The figure shows three views and two pictorial views of one solid part (mm, origin at its lowest corner). Answer the questions. A direction names the side the tool comes from. Coordinates: 2 decimals unless noted, no trailing zeros. Write each loop counter-clockwise with the first axis right and the second up, starting at its lowest first coordinate (ties: lowest second). Pieces come first, ordered by that corner, then holes. Notation, with made-up numbers: (41, 46) - (54, 46) arc R20 ccw to (54, 68) - close; hole circle Ø3 at (16, 4.25). An arc over 180 degrees is marked (long way). Use a Markdown table: item, result. Add a question column.
(1) The part is cut by section B-B, the plane y = 10. Give the vertices of the cut face in (x, z), then the cut area to 3 significant figures.
(2) The part is cut by section D-D, the plane y = 2.75. Give the vertices of the cut face in (x, z), then the cut area to 3 significant figures.
(3) For a pull along X with two mould halves and no side action, classify the marked faces 1, 2 and 3 as released by +X, released by -X, zero draft, split by the parting line, or undercut.
(4) A tool of negligible diameter and unlimited length cuts with its end or side. For the marked faces 4 and 5, from which of +Z, -Z, +X, -X, +Y, -Y can it reach the whole face along a straight path? Write none if from no direction.
(5) Find the intervals of material crossed by line 1 (Y direction, x = 3.5, z = 1.75); line 2 (Y direction, x = 10, z = 1.4); line 3 (X direction, y = 9.25, z = 1.9), in increasing order. Write a range as from..to.
(6) Given pin 1 Ø10 at (x, y) = (6, 12) entering from +Z; pin 2 Ø1 at (y, z) = (14.5, 1.5) entering from -X, each flat-ended and moving along its own axis, determine where each tip first touches the part or whether it passes through.
(7) The part is cut by section A-A, the plane z = 1.75. Give the vertices of the cut face in (x, y).
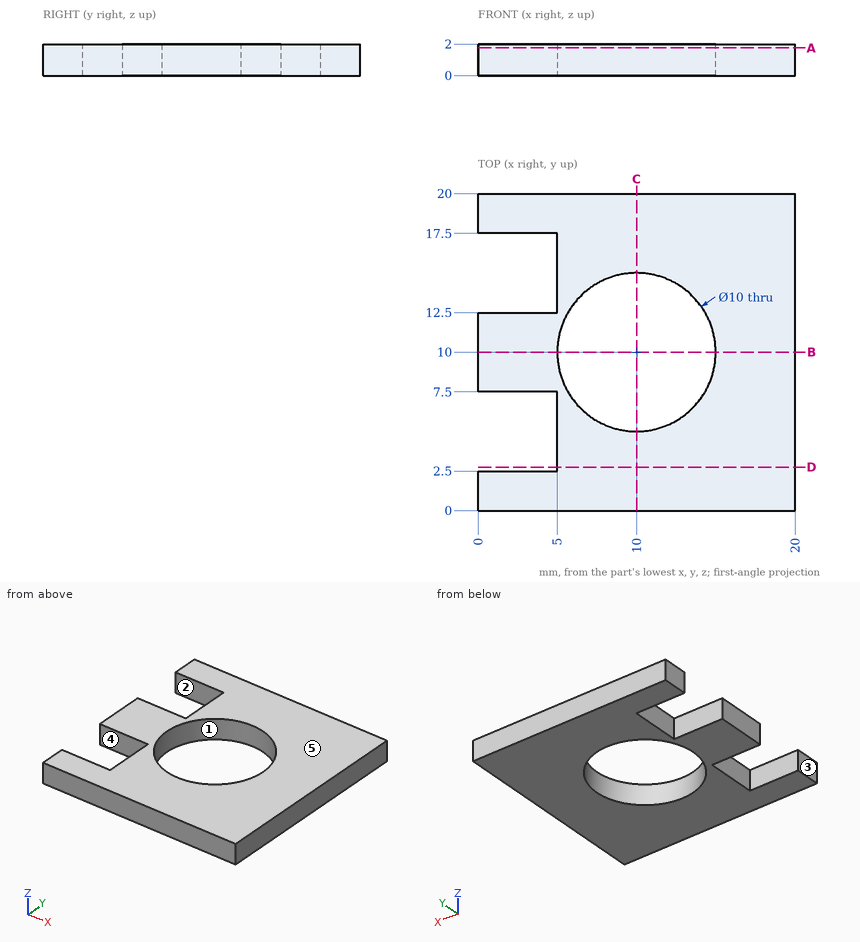
Model answer:
| question | item | result |
|---|---|---|
| 1 | outline | (0, 0) - (5, 0) - (5, 2) - (0, 2) - close; (15, 0) - (20, 0) - (20, 2) - (15, 2) - close |
| 1 | area | 20.0 mm^2 |
| 2 | outline | (5, 0) - (20, 0) - (20, 2) - (5, 2) - close |
| 2 | area | 30.0 mm^2 |
| 3 | face 1 | undercut |
| 3 | face 2 | zero draft |
| 3 | face 3 | released by -X |
| 4 | face 4 | +Z, -Z, -X |
| 4 | face 5 | +Z, +X, -X, +Y, -Y |
| 5 | line 1 | 0..2.5, 7.5..12.5, 17.5..20 |
| 5 | line 2 | 0..5, 15..20 |
| 5 | line 3 | 0..5.06, 14.94..20 |
| 6 | pin 1 | z = 2 |
| 6 | pin 2 | x = 5 |
| 7 | outline | (0, 0) - (20, 0) - (20, 20) - (0, 20) - (0, 17.5) - (5, 17.5) - (5, 12.5) - (0, 12.5) - (0, 7.5) - (5, 7.5) - (5, 2.5) - (0, 2.5) - close; hole circle Ø10 at (10, 10) |
